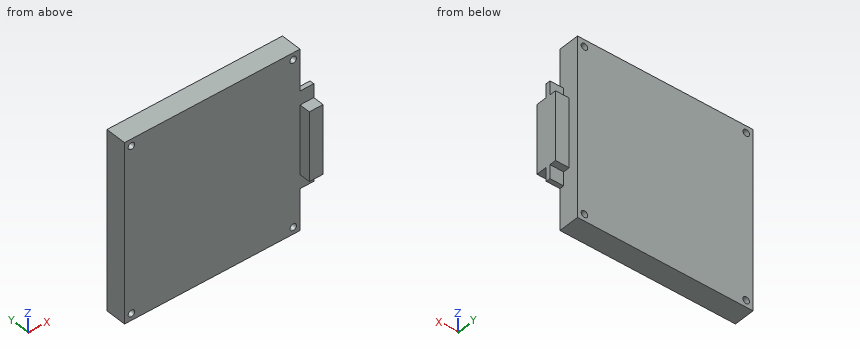
Autodesk Inventor part; units mm, degrees
ref_plane "Work Plane1" through (-64, 0, -32.5) normal (0, 0, 1) x (1, 0, 0)
ref_plane "YZ Plane" through (0, 0, 0) normal (1, 0, 0) x (0, 1, 0)
ref_plane "XZ Plane" through (0, 0, 0) normal (0, 1, 0) x (-1, 0, 0)
sketch "Sketch1" plane through (0, 0, 0) normal (0, 1, 0) x (-1, 0, 0)
  line L0 (0, 0) -> (64, 0)
  line L1 (64, 0) -> (64, -65)
  line L2 (64, -65) -> (0, -65)
  line L3 (0, -65) -> (0, 0)
  line L4 (0, -15) -> (-5, -15)
  line L5 (-5, -15) -> (-5, -50)
  line L6 (-5, -50) -> (0, -50)
  line L7 (0, -50) -> (0, -15)
  dimension "d0" = 64
  dimension "d1" = 65
  dimension "d2" = 5
  dimension "d3" = 15
  dimension "d4" = 15
extrude "Extrusion1" add sketch "Sketch1" along normal blind 1.6
sketch "Sketch2" plane through (0, 0, 0) normal (0, -1, 0) x (1, 0, 0)
  line L0 (5, -15) -> (5, -50)
  line L1 (5, -20) -> (0, -20)
  line L2 (0, -20) -> (0, -45)
  line L3 (0, -45) -> (5, -45)
  line L4 (5, -45) -> (5, -20)
  point P0 (0, 0)
  point P1 (5, -32.5)
  dimension "d7" = 5
  dimension "d8" = 25
extrude "Extrusion2" add sketch "Sketch2" along normal mid plane 8
sketch "Sketch3" plane through (0, 1.6, 0) normal (0, 1, 0) x (1, 0, 0)
  line L0 (0, 0) -> (0, 15)
  line L1 (-64, 65) -> (-64, 0)
  line L2 (0, 0) -> (-64, 0)
  line L3 (-64, 0) -> (-64, 65)
  line L4 (-64, 65) -> (0, 65)
  line L5 (0, 65) -> (0, 0)
extrude "Extrusion3" add sketch "Sketch3" along normal blind 6
sketch "Sketch4" plane through (0, 7.6, 0) normal (0, 1, 0) x (1, 0, 0)
  line L0 (-64, 0) -> (0, 0)
  line L1 (-64, 65) -> (-64, 0)
  point P0 (-61.5, 2.5)
  point P1 (-2.5, 2.5)
  point P2 (-61.5, 62.5)
  point P3 (-2.5, 62.5)
  dimension "d13" = 2.5
  dimension "d14" = 2.5
  dimension "d17" = 59
  dimension "d20" = 60
hole "Hole1" at (-61.5, 7.6, -2.5) at (-2.5, 7.6, -2.5) at (-61.5, 7.6, -62.5) at (-2.5, 7.6, -62.5) direction (0, -1, 0) diameter 2.4 end through all
ref_plane "Work Plane1" through (-64, 0, -32.5) normal (0, 0, 1) x (1, 0, 0)
properties part number "Keypad"
Part model, mm, in its own coordinate system. Coordinates: 2 decimals unless noted, no trailing zeros. Order: outer loops, then holes, each group sorted by start corner. A loop starts at its lowest first (then second) coordinate and runs counter-clockwise, first axis right, second up. Notation, with made-up numbers: (25, 57) - (46, 57) arc R20 ccw to (46, 83) - close; hole circle Ø9 at (67.25, 51). An arc over 180 degrees is marked (long way). Return JSON: item names as keys, results as strings. Group by question number.
Item 1: Cut at C-C (z = -25). List the corners of the cut face in (x, y).
Item 2: Cut at A-A (z = -2.5). List the corners of the cut face in (x, y).
Item 3: Drill centre lines: probe 1 along X at (y, z) = (5.25, -2.5); probe 2 along Z at (x, y) = (-2.5, 4.5); probe 3 along X at (y, z) = (5, -58.5). Where is each one in solid material? Low to high. Write a range as from..to.
Item 4: Pin check, flat tips, straight feed: pin 1 (4 mm diameter, centred on x = -4, y = -3, fed in from -Z); pin 2 (6 mm diameter, centred on x = -18.5, z = -17, fed in from -Y); pin 3 (1.5 mm diameter, centred on x = 3, z = -18.5, fed in from +Y); pin 4 (2 mm diameter, centred on x = 2, y = -2.5, fed in from -Z). Stop position of each tip, or through.
Item 5: Cut at B-B (x = -61.5). List the corners of the cut face in (y, z).
Item 6: Cut at D-D (x = -35.5). List the corners of the cut face in (y, z).
Check values:
{
 "1": {"outline": "(-64, 0) - (0, 0) - (0, -4) - (5, -4) - (5, 4) - (0, 4) - (0, 7.6) - (-64, 7.6) - close"},
 "2": {"outline": "(-64, 0) - (-62.7, 0) - (-62.7, 7.6) - (-64, 7.6) - close; (-60.3, 0) - (-3.7, 0) - (-3.7, 7.6) - (-60.3, 7.6) - close; (-1.3, 0) - (0, 0) - (0, 7.6) - (-1.3, 7.6) - close"},
 "3": {"probe 1": "x = -64..-62.7, -60.3..-3.7, -1.3..0", "probe 2": "z = -65..-63.7, -61.3..-3.7, -1.3..0", "probe 3": "x = -64..0"},
 "4": {"pin 1": "passes through", "pin 2": "stops at y = 0", "pin 3": "stops at y = 1.6", "pin 4": "stops at z = -45"},
 "5": {"outline": "(0, -65) - (7.6, -65) - (7.6, -63.7) - (0, -63.7) - close; (0, -61.3) - (7.6, -61.3) - (7.6, -3.7) - (0, -3.7) - close; (0, -1.3) - (7.6, -1.3) - (7.6, 0) - (0, 0) - close"},
 "6": {"outline": "(0, -65) - (7.6, -65) - (7.6, 0) - (0, 0) - close"}
}
